```python
from build123d import *

# Parameters (mm, degrees)
SKIZZE1_W                       = 40
SKIZZE1_H                       = 3
AUFSATZ_LINEAR_AUSTRAGEN1_DEPTH = 40
VERRUNDUNG1_R                   = 6
SKIZZE2_R                       = 3.5
SCHNITT_LINEAR_AUSTRAGEN1_DEPTH = 10


with BuildPart() as part:
    # Skizze1 → Aufsatz-Linear austragen1 (new, symmetric)
    with BuildSketch(Plane.XY):
        with Locations((0, -1.5)):
            Rectangle(SKIZZE1_W, SKIZZE1_H)
    extrude(amount=AUFSATZ_LINEAR_AUSTRAGEN1_DEPTH, both=True)

    # Verrundung1
    verrundung1_edges = [part.edges().sort_by_distance(p)[0] for p in [
        (20, -1.5, 40),
        (-20, -1.5, 40),
        (20, -1.5, -40),
        (-20, -1.5, -40),
    ]]
    fillet(verrundung1_edges, radius=VERRUNDUNG1_R)

    # Skizze2 → Schnitt-Linear austragen1 (cut)
    with BuildSketch(Plane(origin=(0, 0, 0), x_dir=(1, 0, 0), z_dir=(0, 1, 0))):
        with Locations(Location((6.5, 23, 0), (0, 0, 270))):
            Circle(SKIZZE2_R)
        with Locations(Location((-6.5, 23, 0), (0, 0, 270))):
            Circle(SKIZZE2_R)
        with Locations(Location((6.5, -23, 0), (0, 0, 270))):
            Circle(SKIZZE2_R)
        with Locations(Location((-6.5, -23, 0), (0, 0, 270))):
            Circle(SKIZZE2_R)
    extrude(amount=-SCHNITT_LINEAR_AUSTRAGEN1_DEPTH, mode=Mode.SUBTRACT)


solid = part.part
```
Geometry check sheet. Reference: the model listing, model coordinates, mm. Coordinates: 2 decimals unless noted, no trailing zeros. Loops run counter-clockwise (first coordinate to the right, second up) from the corner with the lowest first, then second, coordinate; pieces in that order, holes last. Notation, with made-up numbers: (76.5, 8.5) -> (127.5, 8.5) arc R34 cw to (127.5, 39.5) -> close; hole circle Ø4 at (42, 42.5). An arc over 180 degrees is marked (long way). Put each result on its own line as item: value.
1) Cross-section at C-C on y = -1.5. Record the boundary of the cut face in (x, z), plus the area to 3 significant figures.
Result set:
outline: (-20, -34) arc R6 ccw to (-14, -40) -> (14, -40) arc R6 ccw to (20, -34) -> (20, 34) arc R6 ccw to (14, 40) -> (-14, 40) arc R6 ccw to (-20, 34) -> close; hole circle Ø7 at (-6.5, -23); hole circle Ø7 at (-6.5, 23); hole circle Ø7 at (6.5, -23); hole circle Ø7 at (6.5, 23)
area: 3,020 mm^2
2) Thickness scan on line 1 (X direction, y = -1.2, z = 23); line 2 (Z direction, x = -6, y = -2.45); line 3 (X direction, y = -2.15, z = 21). Record the ranges inside material, lowest first.
Result set:
line 1: x = -20 to -10, -3 to 3, 10 to 20
line 2: z = -40 to -26.46, -19.54 to 19.54, 26.46 to 40
line 3: x = -20 to -9.37, -3.63 to 3.63, 9.37 to 20
3) Cross-section at B-B on x = -6.5. Record the boundary of the cut face in (y, z), plus the area to 3 significant figures.
Result set:
outline: (-3, -40) -> (0, -40) -> (0, -26.5) -> (-3, -26.5) -> close; (-3, -19.5) -> (0, -19.5) -> (0, 19.5) -> (-3, 19.5) -> close; (-3, 26.5) -> (0, 26.5) -> (0, 40) -> (-3, 40) -> close
area: 198 mm^2
4) Release check for a two-part mould opening along Z. For faces 1 (the flat face through (0, 0, 1)), 2 (the flat face through (0, -1, 40)), 3 (the cylindrical face through (-7.841, -1.479, -19.767)) record: released by +Z, released by -Z, zero draft, split by the parting line, or undercut.
Result set:
face 1: zero draft
face 2: released by +Z
face 3: undercut
5) Cross-section at A-A on z = 23. Record the boundary of the cut face in (x, y), plus the area to 3 significant figures.
Result set:
outline: (-20, -3) -> (-10, -3) -> (-10, 0) -> (-20, 0) -> close; (-3, -3) -> (3, -3) -> (3, 0) -> (-3, 0) -> close; (10, -3) -> (20, -3) -> (20, 0) -> (10, 0) -> close
area: 78.0 mm^2
